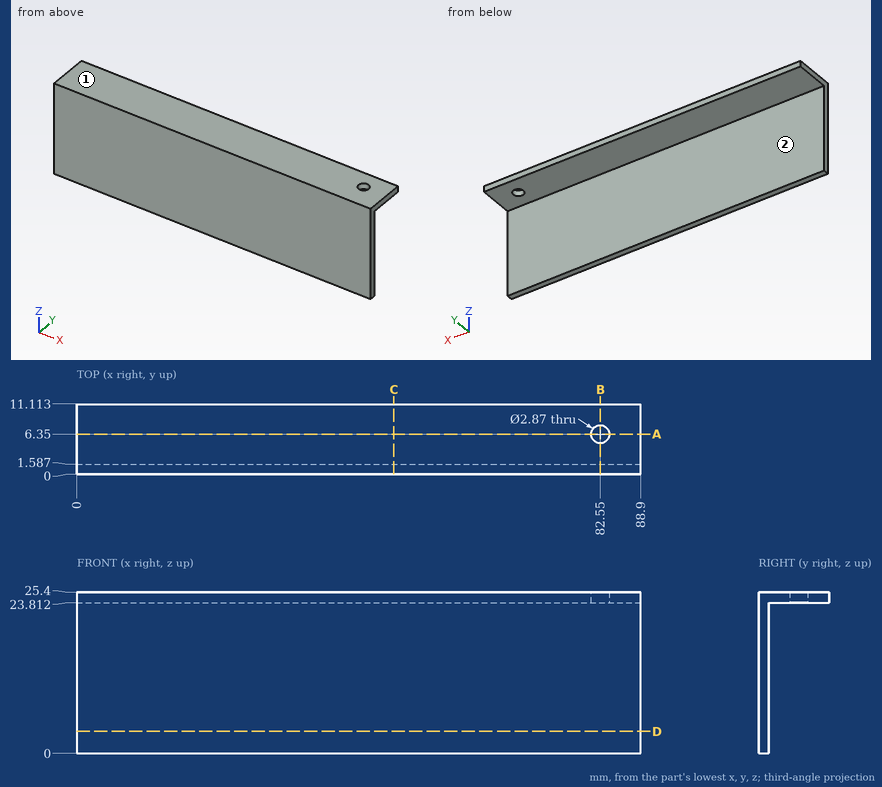
Geometry check sheet. Reference: drawing and pictorial views, mm from the part's lowest x, y, z. A direction names the side the tool comes from. Round coordinates to 2 decimals unless told otherwise and drop trailing zeros. Loops run counter-clockwise (first coordinate to the right, second up) from the corner with the lowest first, then second, coordinate; pieces in that order, holes last. Notation, with made-up numbers: M 5.5,-35.75 L 21.5,-35.75 A11 cw 21.5,-22.75 Z; hole C 52.5,88.5 d5. An arc over 180 degrees is marked long. One line per item, written item: value.
(1) Access from +Z, -Z, +X, -X, +Y, -Y to the whole of each face (thin tool, end or side, straight path). Record for the marked faces 1 and 2.
Computed values:
face 1: +Z, +X, -X, +Y, -Y
face 2: -Z, +X, -X, +Y
(2) Sectioned sample at D-D, the plane z = 3.5. Record the cut outline in (x, y).
Computed values:
outline: M 0,0 L 88.9,0 L 88.9,1.59 L 0,1.59 Z
(3) Thickness scan on line 1 (Y direction, x = 82.55, z = 24.7) (1 decimal); line 2 (Y direction, x = 60, z = 21); line 3 (Z direction, x = 22, y = 10.25). Record the ranges inside material, lowest first.
Computed values:
line 1: y = 0 to 4.9, 7.8 to 11.1
line 2: y = 0 to 1.59
line 3: z = 23.81 to 25.4
(4) Sectioned sample at B-B, the plane x = 82.55. Record the cut outline in (y, z) (1 decimal).
Computed values:
outline: M 0,0 L 1.6,0 L 1.6,23.8 L 4.9,23.8 L 4.9,25.4 L 0,25.4 Z; M 7.8,23.8 L 11.1,23.8 L 11.1,25.4 L 7.8,25.4 Z
(5) Sectioned sample at A-A, the plane y = 6.35. Record the cut outline in (x, z) (1 decimal).
Computed values:
outline: M 0,23.8 L 81.1,23.8 L 81.1,25.4 L 0,25.4 Z; M 84,23.8 L 88.9,23.8 L 88.9,25.4 L 84,25.4 Z
(6) Sectioned sample at C-C, the plane x = 50. Record the cut outline in (y, z).
Computed values:
outline: M 0,0 L 1.59,0 L 1.59,23.81 L 11.11,23.81 L 11.11,25.4 L 0,25.4 Z
(7) Depth check by flat-ended pin: pin 1 Ø1 at (x, z) = (63, 19) entering from +Y. Enter the tip coordinate at first touch or a pass-through.
Computed values:
pin 1: stops at y = 1.59
